For this review, take the finished solid that the model builds, in its own axes (mm). A direction names the side the tool comes from. Coordinates: 2 decimals unless noted, no trailing zeros. Write each loop counter-clockwise with the first axis right and the second up, starting at its lowest first coordinate (ties: lowest second). Pieces come first, ordered by that corner, then holes. Notation, with made-up numbers: M 29,-8.5 L 42,-8.5 A24 ccw 42,24.5 Z; hole C 14.5,78.25 d7. An arc over 180 degrees is marked long. Return JSON: item names as keys, results as strings.
```python
from build123d import *

# Parameters (mm, degrees)
F0_W     = 50
F0_H     = 38
F1_DEPTH = 5
F2_W     = 8
F2_H     = 8
F3_DEPTH = 70
F4_W     = 48
F4_H     = 38
F5_DEPTH = 7


with BuildPart() as f1:
    # F0 (on Front) → F1 (new body)
    with BuildSketch(Plane.XZ):
        Rectangle(F0_W, F0_H)
    extrude(amount=F1_DEPTH)

    # F2 (on Front) → F3 (join)
    with BuildSketch(Plane.XZ):
        with Locations((20.863473, 14.717139)):
            Rectangle(F2_W, F2_H)
        with Locations((20.863473, -14.717139)):
            Rectangle(F2_W, F2_H)
        with Locations((-20.863473, -14.717139)):
            Rectangle(F2_W, F2_H)
        with Locations((-20.863473, 14.717139)):
            Rectangle(F2_W, F2_H)
    extrude(amount=-F3_DEPTH)

    # F4 (on face) → F5 (join)
    with BuildSketch(Plane(origin=(-25, 0, 0), x_dir=(0, -1, 0), z_dir=(-1, 0, 0))):
        with Locations((29, 0)):
            Rectangle(F4_W, F4_H)
    extrude(amount=-F5_DEPTH)


solid = f1.part
```
1. We need section D-D (y = -10). State the section outline as (x, z) points.
Checks:
{"outline": "M -25,-19 L -18,-19 L -18,19 L -25,19 Z"}
2. For faces 5 (the face through (-16.863, 35, -15)), 6 (the face through (-21, 35, -10.717)), 7 (the face through (-24.863, 35, 15)), list the 3-axis set-ups (+Z, -Z, +X, -X, +Y, -Y) from which the entire face can be reached by the end or side of a thin tool; tool diameter is ignored.
Checks:
{"face 5": "+Z, -Z, +Y", "face 6": "+X, -X, +Y", "face 7": "+Z, -Z, -X, +Y"}
3. Clearance check with flat-ended pins moving along their axes: pin 1 Ø11.5 at (x, z) = (-4, 6.5) entering from -Y; pin 2 Ø9 at (x, y) = (-21.5, 18.5) entering from +Z; pin 3 Ø6.5 at (y, z) = (34, -16) entering from +X. State where each tip first meets the part, or that it passes through.
Checks:
{"pin 1": "y = -5", "pin 2": "z = 18.72", "pin 3": "x = 24.86"}
4. We need section A-A (y = 9). State the section outline as (x, z) points, plus the area to 3 significant figures.
Checks:
{"outline": "M -24.86,-18.72 L -16.86,-18.72 L -16.86,-10.72 L -24.86,-10.72 Z; M -24.86,10.72 L -16.86,10.72 L -16.86,18.72 L -24.86,18.72 Z; M 16.86,-18.72 L 24.86,-18.72 L 24.86,-10.72 L 16.86,-10.72 Z; M 16.86,10.72 L 24.86,10.72 L 24.86,18.72 L 16.86,18.72 Z", "area": "256 mm2"}
5. We need section C-C (z = -5). State the section outline as (x, y) points, plus the area to 3 significant figures.
Checks:
{"outline": "M -25,-53 L -18,-53 L -18,-5 L 25,-5 L 25,0 L -25,0 Z", "area": "586 mm2"}
6. Wall thickness on L1, parallel to X at y = 34, z = 17; L2, parallel to Y at x = 11, z = 3; L3, parallel to Y at x = -17.5, z = 11.5: over which ranges is each line inside the solid? List them lowest first. Write a range as from..to.
Checks:
{"L1": "-24.86..-16.86, 16.86..24.86", "L2": "-5..0", "L3": "-5..70"}
7. We need section B-B (x = 22). State the section outline as (y, z) points, plus the area to 3 significant figures.
Checks:
{"outline": "M -5,-19 L 0,-19 L 0,-18.72 L 70,-18.72 L 70,-10.72 L 0,-10.72 L 0,10.72 L 70,10.72 L 70,18.72 L 0,18.72 L 0,19 L -5,19 Z", "area": "1,310 mm2"}
8. Draft analysis for pull direction Z (two halves, no side actions). For faces 1 (the face through (0, 0, 0)), 2 (the face through (16.863, 35, -15)), 3 (the face through (21, 35, 10.717)), 4 (the face through (21, 35, -18.717)), state which applies: +Z half, -Z half, draft (parallel to the pull), parting line (faces both ways), or undercut.
Checks:
{"face 1": "undercut", "face 2": "draft", "face 3": "undercut", "face 4": "-Z half"}
